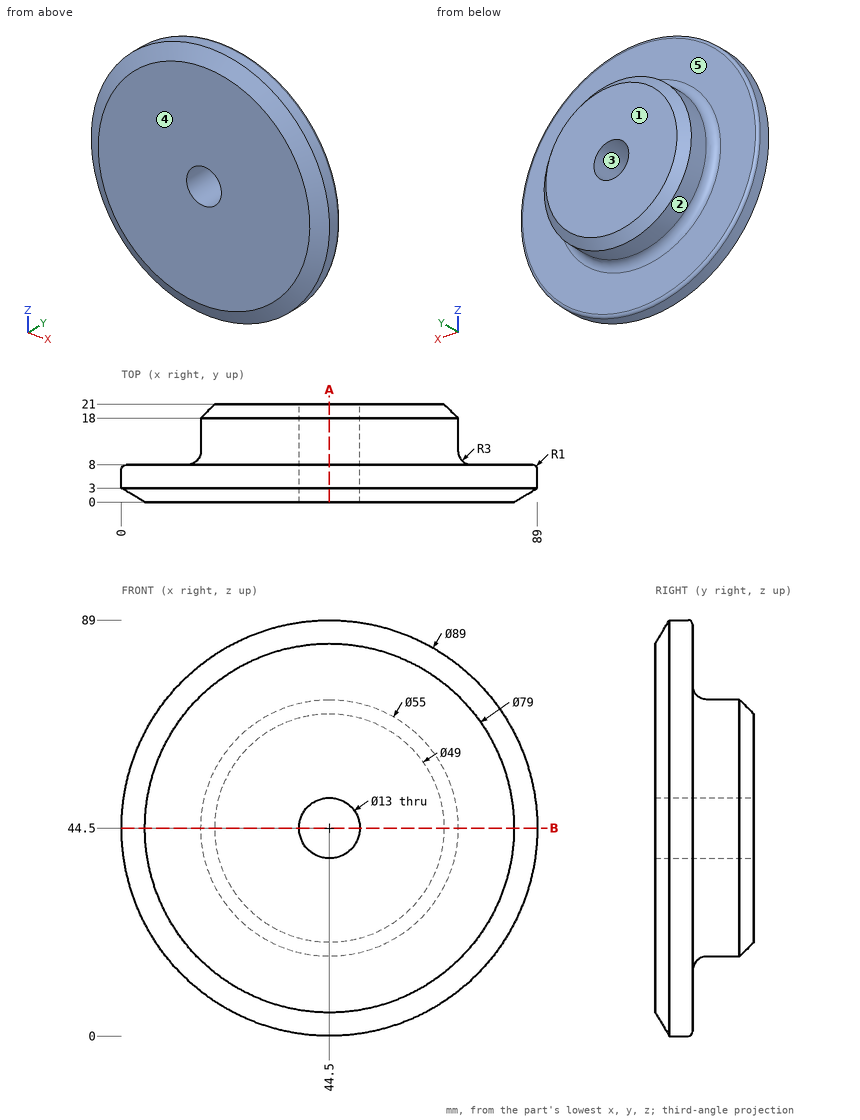
Source: three-view drawing plus pictorial views. Frame: mm from the lowest corner of the part. A direction names the side the tool comes from. Round coordinates to 2 decimals unless told otherwise and drop trailing zeros. Loops run counter-clockwise (first coordinate to the right, second up) from the corner with the lowest first, then second, coordinate; pieces in that order, holes last.
Item 1: Reachability of the marked faces 4 and 5 from +Z, -Z, +X, -X, +Y, -Y: full face, straight path, thin tool, end or side. Return the list, or none.
Checked values:
face 4: +Z, -Z, +X, -X, -Y
face 5: +Y
Item 2: Mould query, pull axis Z, two halves, no side actions, for the marked faces 1, 2 and 3. Classes: released by +Z, released by -Z, zero draft, split by the parting line, or undercut.
Checked values:
face 1: zero draft
face 2: split by the parting line
face 3: undercut
Item 3: Section B-B, the plane z = 44.5. Output: boundary loops of the cut face in (x, y), plus the area to 3 significant figures.
Checked values:
outline: (0, 3) - (5, 0) - (38, 0) - (38, 21) - (20, 21) - (17, 18) - (17, 11) arc R3 cw to (14, 8) - (1, 8) arc R1 ccw to (0, 7) - close; (51, 0) - (84, 0) - (89, 3) - (89, 7) arc R1 ccw to (88, 8) - (75, 8) arc R3 cw to (72, 11) - (72, 18) - (69, 21) - (51, 21) - close
area: 1,130 mm2
Item 4: Line query: L1, parallel to X at y = 13.25, z = 44.5; L2, parallel to X at y = 6, z = 44.5; L3, parallel to Z at x = 44, y = 6.5. Output: solid intervals per line, ascending.
Checked values:
L1: x = 17 to 38, 51 to 72
L2: x = 0 to 38, 51 to 89
L3: z = 0 to 38.02, 50.98 to 89
Item 5: Section A-A, the plane x = 44.5. Output: boundary loops of the cut face in (y, z), plus the area to 3 significant figures.
Checked values:
outline: (0, 5) - (3, 0) - (7, 0) arc R1 ccw to (8, 1) - (8, 14) arc R3 cw to (11, 17) - (18, 17) - (21, 20) - (21, 38) - (0, 38) - close; (0, 51) - (21, 51) - (21, 69) - (18, 72) - (11, 72) arc R3 cw to (8, 75) - (8, 88) arc R1 ccw to (7, 89) - (3, 89) - (0, 84) - close
area: 1,130 mm2
Item 6: Contact query for flat-ended pins moving along their axis: P1, Ø10, axis at y = 18, z = 36, coming from the +X side; P2, Ø1.5, axis at x = 41.5, y = 13, coming from the -Z side; P3, Ø2, axis at x = 66.5, y = 8.5, coming from the -Z side; P4, Ø10.5, axis at x = 44.5, z = 44.5, coming from the +Y side. Output: stop coordinate, or through.
Checked values:
P1: stops at x = 71.78
P2: stops at z = 17.09
P3: stops at z = 5.8
P4: passes through
